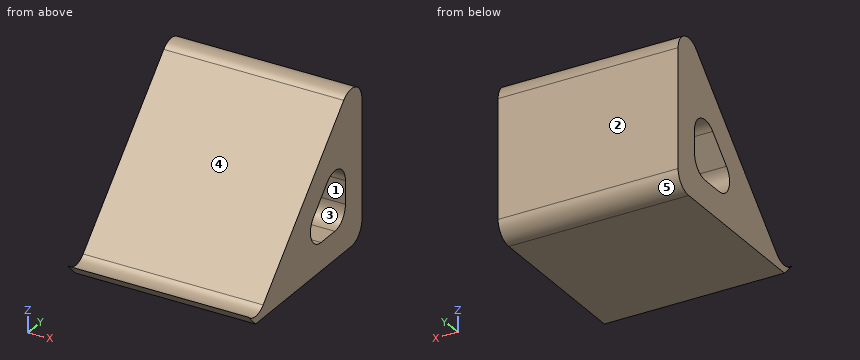
```python
from build123d import *

# Parameters (mm, degrees)
F1_DEPTH = 100
F2_R     = 10


with BuildPart() as f1:
    # F0 (on Right) → F1 (new body)
    with BuildSketch(Plane.YZ):
        Polygon((-50, -50), (50, -50), (50, 50), (-42.928932, -42.928932), align=None)
        Polygon((34.5, -34.5), (-12.57969, -34.5), (34.5, 12.57969), align=None, mode=Mode.SUBTRACT)
        with BuildLine():
            Line((-57.071068, -42.928932), (-50, -50))
            Line((-50, -50), (-42.928932, -42.928932))
            ThreePointArc((-42.928932, -42.928932), (-50, -45.857864), (-57.071068, -42.928932))
        make_face()
    extrude(amount=F1_DEPTH)

    # F2
    f2_edges = [f1.edges().sort_by_distance(p)[0] for p in [
        (50, 50, 50),
        (50, 34.5, 12.57969),
        (50, 50, -50),
        (50, 34.5, -34.5),
        (50, -12.57969, -34.5),
    ]]
    fillet(f2_edges, radius=F2_R)


solid = f1.part
```
Geometry check sheet. Reference: the model listing, model coordinates, mm. Face numbers are marked on the shaded views. A direction names the side the tool comes from. Round coordinates to 2 decimals unless told otherwise and drop trailing zeros. Order: outer loops, then holes, each group sorted by start corner. A loop starts at its lowest first (then second) coordinate and runs counter-clockwise, first axis right, second up. Notation, with made-up numbers: (60, 46) - (109, 46) arc R8 ccw to (109, 55) - close; hole circle Ø1 at (19.5, 78). An arc over 180 degrees is marked (long way). Use a Markdown table: item, result. Add a question column.
1) Section check C-C (z = -21.5). Record the cut outline in (x, y).
2) Section check D-D (z = 12). Record the cut outline in (x, y), then the cut area to 3 significant figures.
3) Mould release check, pull along Z, two halves, no side actions. Record for the marked faces 3, 4 and 5: released by +Z, released by -Z, zero draft, split by the parting line, or undercut.
4) Set-up check for the marked faces 1 and 2: record each of +Z, -Z, +X, -X, +Y, -Y from which the full face is reachable in a straight line by a thin tool's end or side.
5) Section check A-A (x = 89). Record the cut outline in (y, z), then the cut area to 3 significant figures.
6) Section check B-B (y = 21). Record the cut outline in (x, z).
7) Thickness scan on line 1 along Z through (x, y) = (42, 9); line 2 along Z through (x, y) = (10.5, -49.5); line 3 along Z through (x, y) = (7, 13.5). Record the ranges inside material, lowest first.
8) Gauge pin test, flat ends, axial feed: P1, Ø1.5, axis at x = 22, y = -35, coming from the +Z side; P2, Ø10.5, axis at x = 53.5, z = -20, coming from the -Y side; P3, Ø3, axis at x = 18, y = 4.5, coming from the +Z side. Record the tip position at first contact, or that the pin passes through.
Established:
| question | item | result |
|---|---|---|
| 1 | outline | (0, -21.5) - (100, -21.5) - (100, 2.02) - (0, 2.02) - close; (0, 34.5) - (100, 34.5) - (100, 50) - (0, 50) - close |
| 2 | outline | (0, 12) - (100, 12) - (100, 50) - (0, 50) - close |
| 2 | area | 3,800 mm2 |
| 3 | face 3 | undercut |
| 3 | face 4 | released by +Z |
| 3 | face 5 | released by -Z |
| 4 | face 1 | +X, -X |
| 4 | face 2 | +Z, -Z, +X, -X, +Y |
| 5 | outline | (-57.07, -42.93) - (-50, -50) - (40, -50) arc R10 ccw to (50, -40) - (50, 25.86) arc R10 ccw to (32.93, 32.93) - (-42.93, -42.93) arc R10 cw to start; hole (4.49, -17.43) arc R10 ccw to (11.56, -34.5) - (24.5, -34.5) arc R10 ccw to (34.5, -24.5) - (34.5, -11.56) arc R10 ccw to (17.43, -4.49) - close |
| 5 | area | 4,040 mm2 |
| 6 | outline | (0, -50) - (100, -50) - (100, -34.5) - (0, -34.5) - close; (0, -2.19) - (100, -2.19) - (100, 21) - (0, 21) - close |
| 7 | line 1 | -50 to -34.17, -12.92 to 9 |
| 7 | line 2 | -50 to -45.85 |
| 7 | line 3 | -50 to -34.5, -8.42 to 13.5 |
| 8 | P1 | z = -34.25 |
| 8 | P2 | y = -25.25 |
| 8 | P3 | z = 6 |
